```python
from build123d import *

# Parameters (mm, degrees)
SKETCH1_W           = 88.9
SKETCH1_H           = 38.1
BOSS_EXTRUDE1_DEPTH = 6.35
SKETCH2_W           = 88.9
SKETCH2_H           = 6.35
BOSS_EXTRUDE2_DEPTH = 31.75
FILLET1_R           = 2.54
FILLET2_R           = 2.54


with BuildPart() as part:
    # Sketch1 → Boss-Extrude1 (new body)
    with BuildSketch(Plane(origin=(0, 0, 0), x_dir=(1, 0, 0), z_dir=(0, 1, 0))):
        Rectangle(SKETCH1_W, SKETCH1_H)
    extrude(amount=BOSS_EXTRUDE1_DEPTH)

    # Sketch2 → Boss-Extrude2 (add)
    with BuildSketch(Plane(origin=(0, 6.35, 0), x_dir=(1, 0, 0), z_dir=(0, 1, 0))):
        with Locations((0, -15.875)):
            Rectangle(SKETCH2_W, SKETCH2_H)
    extrude(amount=BOSS_EXTRUDE2_DEPTH)

    # Fillet1
    fillet1_edges = [part.edges().sort_by_distance(p)[0] for p in [
        (0, 6.35, 12.7),
    ]]
    fillet(fillet1_edges, radius=FILLET1_R)

    # Fillet2
    fillet2_edges = [part.edges().sort_by_distance(p)[0] for p in [
        (0, 0, 19.05),
    ]]
    fillet(fillet2_edges, radius=FILLET2_R)

    # Sketch3 → CSK for #10 Flat Head Machine Screw (100)1 (revolve, cut)
    with BuildSketch(Plane(origin=(-25.4, 20.32, 19.05), x_dir=(0, -1, 0), z_dir=(1, 0, 0))):
        Polygon((0, 0), (0, 6.35), (4.6101, 6.35), (2.8067, 4.836767725), (2.8067, 1.747676712), (4.8895, 0), align=None)
    revolve(axis=Axis((-25.4, 20.32, 25.4), (0, 0, -1)), mode=Mode.SUBTRACT)

    # Sketch3 at point 2 (carried to point 2, square into its face) → CSK for _10 Flat Head Machine Screw  2 (revolve, cut)
    with BuildSketch(Plane(origin=(25.4, 20.32, 19.05), x_dir=(0, -1, 0), z_dir=(1, 0, 0))):
        Polygon((0, 0), (0, 6.35), (4.6101, 6.35), (2.8067, 4.836767725), (2.8067, 1.747676712), (4.8895, 0), align=None)
    revolve(axis=Axis((25.4, 20.32, 25.4), (0, 0, -1)), mode=Mode.SUBTRACT)

    # Sketch3 at point 3 (carried to point 3, square into its face) → CSK for _10 Flat Head Machine Screw  3 (revolve, cut)
    with BuildSketch(Plane(origin=(33.02, 0, -1.27), x_dir=(0, 0, -1), z_dir=(1, 0, 0))):
        Polygon((0, 0), (0, 6.35), (4.6101, 6.35), (2.8067, 4.836767725), (2.8067, 1.747676712), (4.8895, 0), align=None)
    revolve(axis=Axis((33.02, -6.35, -1.27), (0, 1, 0)), mode=Mode.SUBTRACT)

    # Sketch3 at point 4 (carried to point 4, square into its face) → CSK for _10 Flat Head Machine Screw  4 (revolve, cut)
    with BuildSketch(Plane(origin=(-33.02, 0, -1.27), x_dir=(0, 0, -1), z_dir=(1, 0, 0))):
        Polygon((0, 0), (0, 6.35), (4.6101, 6.35), (2.8067, 4.836767725), (2.8067, 1.747676712), (4.8895, 0), align=None)
    revolve(axis=Axis((-33.02, -6.35, -1.27), (0, 1, 0)), mode=Mode.SUBTRACT)

    # Sketch3 at point 5 (carried to point 5, square into its face) → CSK for _10 Flat Head Machine Screw  5 (revolve, cut)
    with BuildSketch(Plane(origin=(0, 6.35, -1.27), x_dir=(0, 0, 1), z_dir=(1, 0, 0))):
        Polygon((0, 0), (0, 6.35), (4.6101, 6.35), (2.8067, 4.836767725), (2.8067, 1.747676712), (4.8895, 0), align=None)
    revolve(axis=Axis((0, 12.7, -1.27), (0, -1, 0)), mode=Mode.SUBTRACT)


solid = part.part
```
Input: part model. Units: mm. Frame: model coordinates. A direction names the side the tool comes from. Give positions to 0.01 mm unless a question says otherwise; leave off trailing zeros. Loops run counter-clockwise (first coordinate to the right, second up) from the corner with the lowest first, then second, coordinate; pieces in that order, holes last. Notation, with made-up numbers: M -0.75,39 L 29.25,39 A33 cw 29.25,69 Z; hole C 20.5,80 d2. An arc over 180 degrees is marked long. Answer as CSV lines item,"result". Start each with the question number.
1. Section B-B on x = 33.02. Return loops of the section in (y, z), plus the area to 3 significant figures.
2. Line query: L1, parallel to X at y = 20.32, z = 16; L2, parallel to X at y = 2, z = -1; L3, parallel to Z at x = -33, y = 3. Output: solid intervals per line, ascending.
3. Section C-C on x = 17. Return loops of the section in (y, z), plus the area to 3 significant figures.
4. Pin query (flat end, axial travel): P1, Ø6.5, axis at x = 0, z = -1.27, coming from the +Y side; P2, Ø7.5, axis at x = -25.4, y = 20.32, coming from the +Z side; P3, Ø7.5, axis at x = 33.02, z = -1.27, coming from the -Y side. Return the tip coordinate at first contact, or that it passes through.
5. Reachability of faces 1 (the face through (2.867, 4.712, -1.907)), 2 (the face through (-1, 23, 12.7)) from +Z, -Z, +X, -X, +Y, -Y: full face, straight path, thin tool, end or side. Return the list, or none.
6. Section D-D on y = 36. Return loops of the section in (x, z).
7. Section A-A on z = -1.27. Return loops of the section in (x, y).
8. Pull-direction query (Y, two-part tool) for faces 3 (the face through (27.108, 22.547, 15.779)), 4 (the face through (35.626, 1.638, -2.625)), 5 (the face through (22.924, 18.741, 17.412)), 6 (the face through (-1, 6.35, -8)); classes: released by +Y, released by -Y, zero draft, split by the parting line, or undercut.
Computed values:
1,outline,"M 0,-19.05 L 6.35,-19.05 L 6.35,-5.88 L 4.84,-4.08 L 1.75,-4.08 L 0,-6.16 Z; M 0,3.62 L 1.75,1.54 L 4.84,1.54 L 6.35,3.34 L 6.35,10.16 A2.54 cw 8.89,12.7 L 38.1,12.7 L 38.1,19.05 L 2.54,19.05 A2.54 ccw 0,16.51 Z"
1,area,"402 mm²"
2,L1,"x = -44.45 to -28.21, -22.59 to 22.59, 28.21 to 44.45"
2,L2,"x = -44.45 to -35.81, -30.23 to -2.79, 2.79 to 30.23, 35.81 to 44.45"
2,L3,"z = -19.05 to -4.08, 1.54 to 19.05"
3,outline,"M 0,-19.05 L 6.35,-19.05 L 6.35,10.16 A2.54 cw 8.89,12.7 L 38.1,12.7 L 38.1,19.05 L 2.54,19.05 A2.54 ccw 0,16.51 Z"
3,area,"444 mm²"
4,P1,"stops at y = 4.97"
4,P2,"stops at z = 18.09"
4,P3,"stops at y = 0.96"
5,face 1,"+Y"
5,face 2,"-Z, +X, -X, +Y"
6,outline,"M -44.45,12.7 L 44.45,12.7 L 44.45,19.05 L -44.45,19.05 Z"
7,outline,"M -44.45,0 L -37.91,0 L -35.83,1.75 L -35.83,4.84 L -37.63,6.35 L -44.45,6.35 Z; M -30.21,1.75 L -28.13,0 L -4.61,0 L -2.81,1.51 L -2.81,4.6 L -4.89,6.35 L -28.41,6.35 L -30.21,4.84 Z; M 2.81,1.51 L 4.61,0 L 28.13,0 L 30.21,1.75 L 30.21,4.84 L 28.41,6.35 L 4.89,6.35 L 2.81,4.6 Z; M 35.83,1.75 L 37.91,0 L 44.45,0 L 44.45,6.35 L 37.63,6.35 L 35.83,4.84 Z"
8,face 3,"undercut"
8,face 4,"released by -Y"
8,face 5,"undercut"
8,face 6,"released by +Y"
